from build123d import *

# Parameters (mm, degrees)
F0_W     = 20
F0_H     = 50
F0_R     = 5.8996417904
F1_DEPTH = 10
F2_W     = 6.6084070038
F2_H     = 8.3198506385
F3_DEPTH = 25.4
F4_R     = 2.921
F5_R     = 4.9670029832
F6_R     = 0.9909047391
F7_DEPTH = 9.017


with BuildPart() as f1:
    # F0 (on Top) → F1 (new body)
    with BuildSketch(Plane.XY):
        Rectangle(F0_W, F0_H)
        Circle(F0_R, mode=Mode.SUBTRACT)
    extrude(amount=F1_DEPTH)

    # F2 (on face) → F3 (join)
    with BuildSketch(Plane.XY.offset(10)):
        with Locations((-6.6957964981, -20.8400746807)):
            Rectangle(F2_W, F2_H)
    extrude(amount=F3_DEPTH)

    # F4
    f4_edges = [f1.edges().sort_by_distance(p)[0] for p in [
        (-10, -20.840075, 35.4),
        (-6.695796, -25, 35.4),
        (-3.391593, -20.840075, 35.4),
        (-6.695796, -16.680149, 35.4),
    ]]
    fillet(f4_edges, radius=F4_R)

    # F5
    f5_edges = [f1.edges().sort_by_distance(p)[0] for p in [
        (10, 25, 5),
        (-10, 25, 5),
        (0, 25, 0),
        (0, 25, 10),
    ]]
    fillet(f5_edges, radius=F5_R)

    # F6 (on face) → F7 (cut)
    with BuildSketch(Plane.XZ.offset(25)):
        with Locations((-6.9817616604, 24.5982613415)):
            Circle(F6_R)
    extrude(amount=-F7_DEPTH, mode=Mode.SUBTRACT)


solid = f1.part
Geometry: final body of the model. Coordinates: model frame, mm. A direction names the side the tool comes from. Give positions to 0.01 mm unless a question says otherwise; leave off trailing zeros. Write each loop counter-clockwise with the first axis right and the second up, starting at its lowest first coordinate (ties: lowest second). Pieces come first, ordered by that corner, then holes. Notation, with made-up numbers: (70.25, 77) -> (111.25, 77) arc R30 ccw to (111.25, 110) -> close; hole circle Ø1 at (46, 49.5). An arc over 180 degrees is marked (long way). Answer as a JSON object with one key per item and string values.
1. Ray query, probe 1 along Z at (x, y) = (-2.5, -12); probe 2 along Y at (x, z) = (-6.5, 15.5); probe 3 along Z at (x, y) = (-7.5, -22). Return the intervals inside material, ascending. Write a range as from..to.
Ans:
{"probe 1": "z = 0..10", "probe 2": "y = -25..-16.68", "probe 3": "z = 0..23.75, 25.44..35.37"}
2. Cut plane C-C on z = 2.5. Output: boundary loops of the cut face in (x, y), and give its area (3 significant figures).
Ans:
{"outline": "(-10, -25) -> (10, -25) -> (10, 20.03) arc R4.97 ccw to (7.5, 24.34) -> (-7.5, 24.34) arc R4.97 ccw to (-10, 20.03) -> close; hole circle Ø11.8 at (0, 0)", "area": "871 mm^2"}
3. Access query for faces 4 (the flat face through (-7, -16.68, 21)), 5 (the cylindrical face through (-9.13, 22.84, 5.07)), 6 (the flat face through (-3.392, -21, 21)). Directions: +Z, -Z, +X, -X, +Y, -Y. A direction counts if a zero-diameter tool reaches every point of the face in a straight line with its end or side. Return the directions, or none.
Ans:
{"face 4": "+Z, +X, -X, +Y", "face 5": "+Z, -Z, -X, +Y", "face 6": "+Z, +X, +Y, -Y"}
4. Cut plane A-A on x = 0. Output: boundary loops of the cut face in (y, z).
Ans:
{"outline": "(-25, 0) -> (-5.9, 0) -> (-5.9, 10) -> (-25, 10) -> close; (5.9, 0) -> (20.03, 0) arc R4.97 ccw to (25, 4.97) -> (25, 5.03) arc R4.97 ccw to (20.03, 10) -> (5.9, 10) -> close"}
5. Cut plane D-D on y = -21. Output: boundary loops of the cut face in (x, z).
Ans:
{"outline": "(-10, 0) -> (10, 0) -> (10, 10) -> (-3.39, 10) -> (-3.39, 32.48) arc R2.92 ccw to (-6.31, 35.4) -> (-7.08, 35.4) arc R2.92 ccw to (-10, 32.48) -> close; hole circle Ø1.98 at (-6.98, 24.6)"}
6. Cut plane B-B on y = 0. Output: boundary loops of the cut face in (x, z), and give its area (3 significant figures).
Ans:
{"outline": "(-10, 0) -> (-5.9, 0) -> (-5.9, 10) -> (-10, 10) -> close; (5.9, 0) -> (10, 0) -> (10, 10) -> (5.9, 10) -> close", "area": "82.0 mm^2"}
7. Contact query for flat-ended pins moving along their axis: pin 1 (1 mm diameter, centred on x = 1, y = 13, fed in from +Z); pin 2 (2 mm diameter, centred on x = -6, z = 26.5, fed in from +Y); pin 3 (4 mm diameter, centred on y = -21, z = 21, fed in from +X). Output: stop coordinate, or through.
Ans:
{"pin 1": "stops at z = 10", "pin 2": "stops at y = -16.68", "pin 3": "stops at x = -3.39"}
8. Mould query, pull axis Y, two halves, no side actions, for faces 1 (the cylindrical face through (5.627, 1.772, 4.93)), 2 (the cylindrical face through (0.14, 22.84, 0.87)), 3 (the cylindrical face through (-6.52, -20.9, 23.72)). Classes: pulls with the +Y half, pulls with the -Y half, needs draft (parallel to the pull), parting line crosses it, or undercut.
Ans:
{"face 1": "undercut", "face 2": "pulls with the +Y half", "face 3": "needs draft"}
